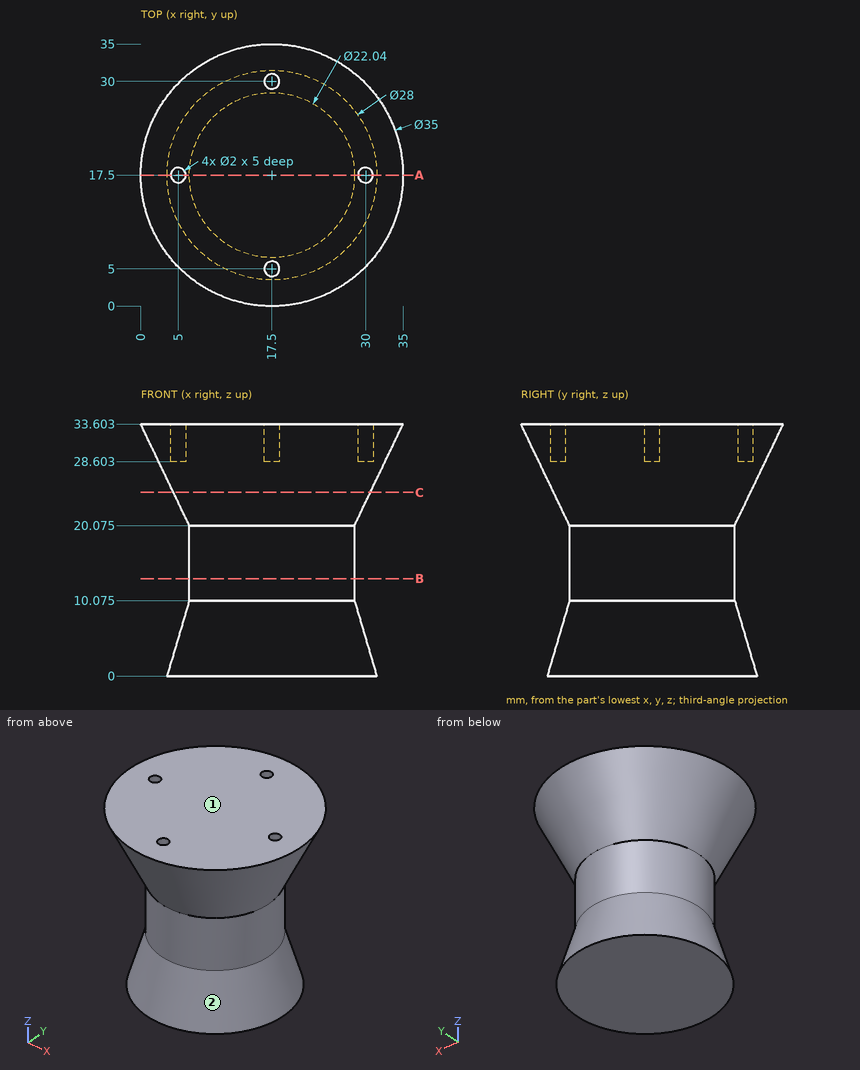
Could you check a few things on this drawing? It's one solid part, dimensions in mm from its lowest x, y, z. A direction names the side the tool comes from. Round coordinates to 2 decimals unless told otherwise and drop trailing zeros. Loops run counter-clockwise (first coordinate to the right, second up) from the corner with the lowest first, then second, coordinate; pieces in that order, holes last.
Q1. Please list where these lines run through material, in increasing order: L1, parallel to Y at x = 17.5, z = 29.7; L2, parallel to Y at x = 17.5, z = 31.9 (1 decimal); L3, parallel to X at y = 17, z = 15.
Q2. I want a section at C-C (z = 24.5). Write out the boundary of the cut face in (x, y).
Q3. I want a section at B-B (z = 13). Write out the boundary of the cut face in (x, y).
Q4. For P1, Ø1.6, axis at x = 17.5, y = 30, coming from the +Z side; P2, Ø1.5, axis at y = 27, z = 13.5, coming from the -X side; P3, Ø3, axis at x = 20, z = 14.5, coming from the +Y side (1 decimal), each with a flat end and sliding along its axis, tell me the tip position at first contact or that it passes through.
Q5. I want a section at A-A (y = 17.5). Write out the boundary of the cut face in (x, z) (1 decimal), and give its area (3 significant figures).
Q6. On a 3-axis mill with a long thin cutter (end or side, diameter ignored), from which of +Z, -Z, +X, -X, +Y, -Y can I reach the whole of each face in a straight line? I mean the marked faces 1 and 2. Say none if no direction works.
Answer below:
1. L1: y = 1.87 to 4, 6 to 29, 31 to 33.13
1. L2: y = 0.8 to 4, 6 to 29, 31 to 34.2
1. L3: x = 6.49 to 28.51
2. outline: circle Ø26.28 at (17.5, 17.5)
3. outline: circle Ø22.04 at (17.5, 17.5)
4. P1: stops at z = 28.6
4. P2: stops at x = 10.8
4. P3: stops at y = 28.5
5. outline: (0, 33.6) - (6.5, 20.1) - (6.5, 10.1) - (3.5, 0) - (31.5, 0) - (28.5, 10.1) - (28.5, 20.1) - (35, 33.6) - (31, 33.6) - (31, 28.6) - (29, 28.6) - (29, 33.6) - (6, 33.6) - (6, 28.6) - (4, 28.6) - (4, 33.6) - close
5. area: 838 mm2
6. face 1: +Z, +X, -X, +Y, -Y
6. face 2: none
